Geometry check sheet. Reference: the model listing, model coordinates, mm. A direction names the side the tool comes from. Round coordinates to 2 decimals unless told otherwise and drop trailing zeros. Order: outer loops, then holes, each group sorted by start corner. A loop starts at its lowest first (then second) coordinate and runs counter-clockwise, first axis right, second up. Notation, with made-up numbers: M 10,-16.5 L 14,-16.5 A22 ccw 14,18.5 Z; hole C 27,73 d9. An arc over 180 degrees is marked long. Return JSON: item names as keys, results as strings. Group by question number.
Autodesk Fusion 360 part; units mm, degrees
sketch "Sketch1" plane through (0, 0, 0) normal (0, 0, 1) x (1, 0, 0)
  circle A0 centre (0, 0) radius 19
  line L0 (0, 0) -> (0, 68.0684) construction
  line L1 (-12.5, 21.6506) -> (-12.5, 50)
  line L2 (-18.5, 50) -> (-12.5, 50)
  line L3 (12.5, 50) -> (18.5, 50)
  line L4 (-18.5, 50) -> (-18.5, 16.8152)
  line L5 (12.5, 21.6506) -> (12.5, 50)
  line L6 (18.5, 50) -> (18.5, 16.8152)
  arc A1 (-18.5, 16.8152) -> (18.5, 16.8152) centre (0, 0) ccw
  arc A2 (12.5, 21.6506) -> (-12.5, 21.6506) centre (0, 0) ccw
  dimension "d1" = 38
  dimension "d3" = 12.5
  dimension "d5" = 6
extrude "Extrude1" add sketch "Sketch1" along normal blind 15
fillet "Fillet1" radius 20 1 edges at (-18.5, 16.8152, 7.5)
fillet "Fillet2" radius 20 1 edges at (18.5, 16.8152, 7.5)
fillet "Fillet3" radius 5 1 edges at (-12.5, 21.6506, 7.5)
fillet "Fillet4" radius 5 1 edges at (12.5, 21.6506, 7.5)
sketch "Sketch2" plane through (18.5, 0, 0) normal (1, 0, 0) x (0, 1, 0)
  line L0 (23.297, 15) -> (23.297, 0)
  line L1 (23.297, 0) -> (50, 0)
  line L2 (50, 0) -> (50, 15)
  line L3 (50, 15) -> (23.297, 15)
  point P0 (40, 7.5)
  dimension "d17" = 7.5
  dimension "d18" = 10
hole "Hole1" at (18.5, 40, 7.5) direction (-1, 0, 0) diameter 6 depth 70 tip angle 118
fillet "Fillet5" radius 7.5 2 edges at (15.5, 50, 15) (-15.5, 50, 15)
Q1. Section check A-A on y = 0. Record the cut outline in (x, z).
Q2. Material ranges on line 1 along X through (y, z) = (32, 13.5); line 2 along X through (y, z) = (-0.5, 5); line 3 along Z through (x, y) = (-16.1, 40), recorded low to high.
Q3. Release check for a two-part mould opening along X. For faces 6 (the face through (-19.256, 17.849, 7.605)), 7 (the face through (-10.61, 25.13, 7.6)), 8 (the face through (19.215, 17.996, 7.605)), 9 (the face through (-16, 50, 4)) record: +X half, -X half, draft (parallel to the pull), parting line (faces both ways), or undercut.
Q4. Section check B-B on x = -15. Record the cut outline in (y, z).
Q5. Depth check by flat-ended pin: pin 1 Ø12 at (x, y) = (-2, 28) entering from +Z; pin 2 Ø7 at (y, z) = (40, 7.5) entering from +X; pin 3 Ø1 at (x, z) = (18.5, 2) entering from -Y; pin 4 Ø1 at (x, y) = (17, 2) entering from -Z (3 decimals). Enter the tip coordinate at first touch or a pass-through.
Q6. Section check D-D on z = 2. Record the cut outline in (x, y), plus the area to 3 significant figures.
Q7. Set-up check for faces 1 (the face through (18.5, 36.8, 7.4)), 2 (the face through (-15.458, 47.861, 12.745)), 3 (the face through (-18.5, 36.8, 7.4)), 4 (the face through (8.767, 16.856, 7.395)), 5 (the face through (12.5, 37, 6)): record each of +Z, -Z, +X, -X, +Y, -Y from which the full face is reachable in a straight line by a thin tool's end or side.
Geometry check:
{
 "1": {"outline": "M -25,0 L -19,0 L -19,15 L -25,15 Z; M 19,0 L 25,0 L 25,15 L 19,15 Z"},
 "2": {"line 1": "x = -18.5 to -12.5, 12.5 to 18.5", "line 2": "x = -25 to -18.99, 18.99 to 25", "line 3": "z = 0 to 4.5, 10.5 to 15"},
 "3": {"face 6": "-X half", "face 7": "undercut", "face 8": "+X half", "face 9": "draft"},
 "4": {"outline": "M -20,0 L -11.66,0 L -11.66,15 L -20,15 Z; M 11.66,0 L 50,0 L 50,7.5 A7.5 ccw 42.5,15 L 11.66,15 Z; hole C 40,7.5 d6"},
 "5": {"pin 1": "stops at z = 15", "pin 2": "stops at x = 18.5", "pin 3": "stops at y = -17.35", "pin 4": "passes through"},
 "6": {"outline": "M -21.39,12.94 A25 ccw long 21.39,12.94 A20 cw 18.5,23.3 L 18.5,50 L 12.5,50 L 12.5,29.05 A5 cw 6.25,24.21 A25 ccw -6.25,24.21 A5 cw -12.5,29.05 L -12.5,50 L -18.5,50 L -18.5,23.3 A20 cw Z; hole C 0,0 d38", "area": "1,230 mm^2"},
 "7": {"face 1": "+Z, -Z, +X, +Y", "face 2": "+Z, +X, -X, +Y", "face 3": "+Z, -Z, -X, +Y", "face 4": "+Z, -Z", "face 5": "+Z, -Z, +Y"}
}
